```python
from build123d import *

# Parameters (mm, degrees)
SKETCH1_R           = 1.4605
SKETCH1_R_2         = 5.08
BOSS_EXTRUDE1_DEPTH = 1.524


with BuildPart() as part:
    # Sketch1 → Boss-Extrude1 (new body)
    with BuildSketch(Plane(origin=(0, 0, 0), x_dir=(1, 0, 0), z_dir=(0, 1, 0))):
        with BuildLine():
            Line((-90.551, 0), (-9.906, 0))
            ThreePointArc((-9.906, 0), (-3.398484286, 2.396683595), (0, 8.441694561))
            Line((0, 8.441694561), (0, 11.624305439))
            ThreePointArc((0, 11.624305439), (-3.398484286, 17.669316405), (-9.906, 20.066))
            Line((-9.906, 20.066), (-90.551, 20.066))
            Line((-90.551, 20.066), (-90.551, 0))
        make_face()
        with Locations(Location((-69.469, 3.556, 0), (0, 0, 90))):
            Circle(SKETCH1_R, mode=Mode.SUBTRACT)
        with Locations(Location((-49.53, 3.556, 0), (0, 0, 90))):
            Circle(SKETCH1_R, mode=Mode.SUBTRACT)
        with Locations(Location((-29.591, 3.556, 0), (0, 0, 90))):
            Circle(SKETCH1_R, mode=Mode.SUBTRACT)
        with Locations(Location((-69.469, 16.51, 0), (0, 0, 90))):
            Circle(SKETCH1_R, mode=Mode.SUBTRACT)
        with Locations(Location((-49.53, 16.51, 0), (0, 0, 90))):
            Circle(SKETCH1_R, mode=Mode.SUBTRACT)
        with Locations(Location((-9.906, 10.033, 0), (0, 0, 90))):
            Circle(SKETCH1_R_2, mode=Mode.SUBTRACT)
        with Locations(Location((-29.591, 16.51, 0), (0, 0, 90))):
            Circle(SKETCH1_R, mode=Mode.SUBTRACT)
    extrude(amount=BOSS_EXTRUDE1_DEPTH)


solid = part.part
```
Verification items for the finished model (mm, model axes). Coordinates: 2 decimals unless noted, no trailing zeros. Write each loop counter-clockwise with the first axis right and the second up, starting at its lowest first coordinate (ties: lowest second). Pieces come first, ordered by that corner, then holes. Notation, with made-up numbers: M 2.5,41 L 6.5,41 A5 cw 6.5,45 Z; hole C 88,72.5 d9. An arc over 180 degrees is marked long. Answer as a JSON object with one key per item and string values. Group by question number.
(1) Release check for a two-part mould opening along Z. For faces 1 (the face through (-68.043, 0.751, -3.239)), 2 (the face through (-3.32, 0.75, -17.6)), 3 (the face through (-46, 0, -10)) record: +Z half, -Z half, draft (parallel to the pull), parting line (faces both ways), or undercut.
(2) Cross-section at B-B, the plane z = -10.25. Record the cut outline in (x, y), and give its area (3 significant figures).
(3) Material ranges on line 1 (Z direction, x = -49.5, y = 1.4); line 2 (X direction, y = 0.5, z = -16.5); line 3 (X direction, y = 1.4, z = -2.75), recorded low to high.
(4) Cross-section at C-C, the plane y = 1.05. Record the cut outline in (x, z), and give its area (3 significant figures).
(5) Cross-section at A-A, the plane x = -49.53. Record the cut outline in (y, z), and give its area (3 significant figures).
(6) Cross-section at D-D, the plane z = -16.51. Record the cut outline in (x, y).
(7) Gauge pin test, flat ends, axial feed: pin 1 (2.5 mm diameter, centred on x = -69.469, z = -16.51, fed in from -Y); pin 2 (5 mm diameter, centred on x = -19.5, z = -15.5, fed in from -Y). Record the tip position at first contact, or that the pin passes through.
Reply:
{
 "1": {"face 1": "undercut", "face 2": "-Z half", "face 3": "draft"},
 "2": {"outline": "M -90.55,0 L -14.98,0 L -14.98,1.52 L -90.55,1.52 Z; M -4.83,0 L 0,0 L 0,1.52 L -4.83,1.52 Z", "area": "123 mm²"},
 "3": {"line 1": "-20.07 to -17.97, -15.05 to -5.02, -2.1 to 0", "line 2": "-90.55 to -70.93, -68.01 to -50.99, -48.07 to -31.05, -28.13 to -2.24", "line 3": "-90.55 to -70.69, -68.25 to -50.75, -48.31 to -30.81, -28.37 to -3.01"},
 "4": {"outline": "M -90.55,-20.07 L -9.91,-20.07 A10.03 ccw 0,-11.62 L 0,-8.44 A10.03 ccw -9.91,0 L -90.55,0 Z; hole C -69.47,-16.51 d2.92; hole C -69.47,-3.56 d2.92; hole C -49.53,-16.51 d2.92; hole C -49.53,-3.56 d2.92; hole C -29.59,-16.51 d2.92; hole C -29.59,-3.56 d2.92; hole C -9.91,-10.03 d10.16", "area": "1,650 mm²"},
 "5": {"outline": "M 0,-20.07 L 1.52,-20.07 L 1.52,-17.97 L 0,-17.97 Z; M 0,-15.05 L 1.52,-15.05 L 1.52,-5.02 L 0,-5.02 Z; M 0,-2.1 L 1.52,-2.1 L 1.52,0 L 0,0 Z", "area": "21.7 mm²"},
 "6": {"outline": "M -90.55,0 L -70.93,0 L -70.93,1.52 L -90.55,1.52 Z; M -68.01,0 L -50.99,0 L -50.99,1.52 L -68.01,1.52 Z; M -48.07,0 L -31.05,0 L -31.05,1.52 L -48.07,1.52 Z; M -28.13,0 L -2.24,0 L -2.24,1.52 L -28.13,1.52 Z"},
 "7": {"pin 1": "through", "pin 2": "y = 0"}
}
